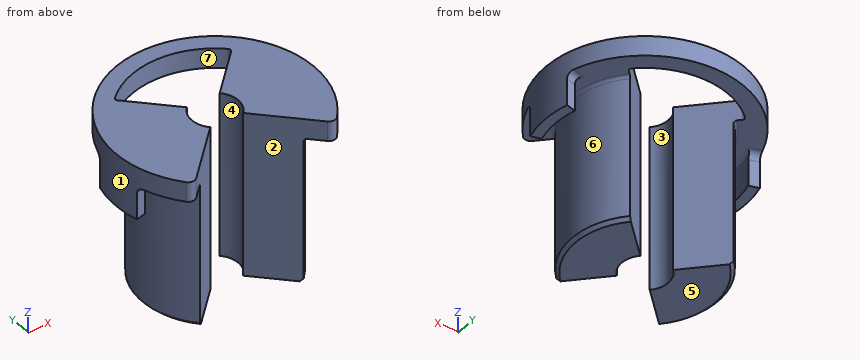
from build123d import *

# Parameters (mm, degrees)
F0_R      = 11
F0_R_2    = 3.5
F1_DEPTH  = 25
F2_R      = 15
F2_R_2    = 3.5
F3_DEPTH  = 8
F4_R      = 13.5
F4_R_2    = 11
F5_DEPTH  = 5
F6_R      = 0.4
F8_DEPTH  = 25
F10_DEPTH = 5
F12_R     = 1
F13_SIZE  = 0.5
F15_DEPTH = 3
F16_R     = 0.4


# Not quite as in the source:
# - a feature of the source that left no trace in its solid (it failed there, or was rolled back) is left out


with BuildPart() as f1:
    # F0 (on Top) → F1 (new body)
    with BuildSketch(Plane.XY):
        Circle(F0_R)
        Circle(F0_R_2, mode=Mode.SUBTRACT)
    extrude(amount=-F1_DEPTH)

    # F2 (on Top) → F3 (join)
    with BuildSketch(Plane.XY):
        Circle(F2_R)
        Circle(F2_R_2, mode=Mode.SUBTRACT)
    extrude(amount=-F3_DEPTH)

    # F4 (on face) → F5 (cut)
    with BuildSketch(Plane(origin=(0, 0, -8), x_dir=(1, 0, 0), z_dir=(0, 0, -1))):
        Circle(F4_R)
        Circle(F4_R_2, mode=Mode.SUBTRACT)
    extrude(amount=-F5_DEPTH, mode=Mode.SUBTRACT)

    # F6
    f6_edges = [f1.edges().sort_by_distance(p)[0] for p in [
        (-13.5, 0, -3),
    ]]
    fillet(f6_edges, radius=F6_R)

    # F7 (on Top) → F8 (cut)
    with BuildSketch(Plane.XY):
        with BuildLine():
            ThreePointArc((-2.4748737342, 2.4748737342), (0, 3.5), (2.4748737342, 2.4748737342))
            Line((2.4748737342, 2.4748737342), (10.6066017178, 10.6066017178))
            ThreePointArc((10.6066017178, 10.6066017178), (0, 15), (-10.6066017178, 10.6066017178))
            Line((-10.6066017178, 10.6066017178), (-2.4748737342, 2.4748737342))
        make_face()
        with BuildLine():
            Line((10.6066017178, -10.6066017178), (2.4748737342, -2.4748737342))
            ThreePointArc((2.4748737342, -2.4748737342), (0, -3.5), (-2.4748737342, -2.4748737342))
            Line((-2.4748737342, -2.4748737342), (-10.6066017178, -10.6066017178))
            ThreePointArc((-10.6066017178, -10.6066017178), (0, -15), (10.6066017178, -10.6066017178))
        make_face()
    extrude(amount=-F8_DEPTH, mode=Mode.SUBTRACT)

    # F9 (on face) → F10 (cut, through all)
    with BuildSketch(Plane(origin=(0, 0, -8), x_dir=(1, 0, 0), z_dir=(0, 0, -1))):
        with BuildLine():
            ThreePointArc((-10.6251840892, 2.8470094961), (0, 11), (10.6251840892, 2.8470094961))
            Line((10.6251840892, 2.8470094961), (15.4548132206, 4.1411047216))
            ThreePointArc((15.4548132206, 4.1411047216), (0, 16), (-15.4548132206, 4.1411047216))
            Line((-15.4548132206, 4.1411047216), (-10.6251840892, 2.8470094961))
        make_face()
        with BuildLine():
            Line((15.4548132206, -4.1411047216), (10.6251840892, -2.8470094961))
            ThreePointArc((10.6251840892, -2.8470094961), (0, -11), (-10.6251840892, -2.8470094961))
            Line((-10.6251840892, -2.8470094961), (-15.4548132206, -4.1411047216))
            ThreePointArc((-15.4548132206, -4.1411047216), (0, -16), (15.4548132206, -4.1411047216))
        make_face()
    extrude(amount=-F10_DEPTH, mode=Mode.SUBTRACT)

    # F12 (call 1 of 6: OpenCascade refuses the feature's edges together)
    f12_edges = [f1.edges().sort_by_distance(p)[0] for p in [
        (10.606602, -10.606602, -1.5),
    ]]
    fillet(f12_edges, radius=F12_R)

    # F12#2 (call 2 of 6)
    f12_2_edges = [f1.edges().sort_by_distance(p)[0] for p in [
        (-10.606602, -10.606602, -1.5),
    ]]
    fillet(f12_2_edges, radius=F12_R)

    # F12#3 (call 3 of 6)
    f12_3_edges = [f1.edges().sort_by_distance(p)[0] for p in [
        (13.571258, -3.636408, -3),
    ]]
    fillet(f12_3_edges, radius=F12_R)

    # F12#4 (call 4 of 6)
    f12_4_edges = [f1.edges().sort_by_distance(p)[0] for p in [
        (13.571258, 3.636408, -3),
    ]]
    fillet(f12_4_edges, radius=F12_R)

    # F12#5 (call 5 of 6)
    f12_5_edges = [f1.edges().sort_by_distance(p)[0] for p in [
        (-13.571258, -3.636408, -3),
    ]]
    fillet(f12_5_edges, radius=F12_R)

    # F12#6 (call 6 of 6)
    f12_6_edges = [f1.edges().sort_by_distance(p)[0] for p in [
        (-13.571258, 3.636408, -3),
    ]]
    fillet(f12_6_edges, radius=F12_R)

    # F13
    f13_edges = [f1.edges().sort_by_distance(p)[0] for p in [
        (-11, 0, -25),
        (11, 0, -25),
    ]]
    chamfer(f13_edges, length=F13_SIZE)

    # F14 (on Top) → F15 (join)
    with BuildSketch(Plane.XY):
        with BuildLine():
            Line((12.5, 0), (15, 0))
            ThreePointArc((15, 0), (0, 15), (-15, 0))
            Line((-15, 0), (-12.5, 0))
            ThreePointArc((-12.5, 0), (0, 12.5), (12.5, 0))
        make_face()
    extrude(amount=-F15_DEPTH)

    # F16
    f16_edges = [f1.edges().sort_by_distance(p)[0] for p in [
        (11, 0, -3),
        (-11, 0, -3),
        (-8.838835, 8.838835, -1.5),
        (8.838835, 8.838835, -1.5),
    ]]
    fillet(f16_edges, radius=F16_R)


solid = f1.part
Build history of the part. All positions in model axes, mm. Face numbers are marked on the shaded views. A direction names the side the tool comes from. Round coordinates to 2 decimals unless told otherwise and drop trailing zeros. Write each loop counter-clockwise with the first axis right and the second up, starting at its lowest first coordinate (ties: lowest second). Pieces come first, ordered by that corner, then holes. Notation, with made-up numbers: M -5,3 L 12,3 A30 cw 12,42 Z; hole C 88,-29.5 d9. An arc over 180 degrees is marked long. Answer in a Markdown table with one row per item.
1. Saw through at B-B (z = -19.5). List the corners of the cut face in (x, y).
Geometry check:
| item | result |
|---|---|
| outline | M -7.78,-7.78 L -2.47,-2.47 A3.5 cw -2.47,2.47 L -7.78,7.78 A11 ccw Z; M 2.47,-2.47 L 7.78,-7.78 A11 ccw 7.78,7.78 L 2.47,2.47 A3.5 cw Z |
2. Saw through at A-A (z = -6.25). List the corners of the cut face in (x, y), and give its area (3 significant figures).
Geometry check:
| item | result |
|---|---|
| outline | M -14.49,-3.88 L -13.04,-3.49 A13.5 cw -13.04,3.49 L -14.49,3.88 A15 ccw Z; M -7.78,-7.78 L -2.47,-2.47 A3.5 cw -2.47,2.47 L -7.78,7.78 A11 ccw Z; M 2.47,-2.47 L 7.78,-7.78 A11 ccw 7.78,7.78 L 2.47,2.47 A3.5 cw Z; M 13.04,-3.49 L 14.49,-3.88 A15 ccw 14.49,3.88 L 13.04,3.49 A13.5 cw Z |
| area | 193 mm2 |
3. Mould opens along Y. For the marked faces 1, 2, 3 and 4 say: +Y half, -Y half, draft (parallel to the pull), parting line (faces both ways), or undercut.
Geometry check:
| item | result |
|---|---|
| face 1 | parting line |
| face 2 | -Y half |
| face 3 | undercut |
| face 4 | undercut |
4. Flat gauge pins, fed straight in: P1, Ø4, axis at x = -0.5, y = 4.5, coming from the -Z side; P2, Ø12, axis at x = 9, z = -20.5, coming from the +Y side; P3, Ø2, axis at x = 5, z = -13.5, coming from the +Y side; P4, Ø2, axis at x = 14.5, y = 0.5, coming from the -Z side. Where does each tip first touch, or does it go through?
Geometry check:
| item | result |
|---|---|
| P1 | through |
| P2 | y = 7.78 |
| P3 | y = 6 |
| P4 | z = -8 |
5. Saw through at C-C (y = 0). List the corners of the cut face in (x, z), and give its area (3 significant figures).
Geometry check:
| item | result |
|---|---|
| outline | M -15,-8 L -13.5,-8 L -13.5,-3.4 A0.4 cw -13.1,-3 L -11.4,-3 A0.4 cw -11,-3.4 L -11,-24.5 L -10.5,-25 L -3.5,-25 L -3.5,0 L -15,0 Z; M 3.5,-25 L 10.5,-25 L 11,-24.5 L 11,-3.4 A0.4 cw 11.4,-3 L 13.1,-3 A0.4 cw 13.5,-3.4 L 13.5,-8 L 15,-8 L 15,0 L 3.5,0 Z |
| area | 414 mm2 |
6. Which spindle directions (+Z, -Z, +X, -X, +Y, -Y) get a long thin tool onto all of the face, cutting with end or side? Do the marked faces 5, 6 and 7. Say none if no direction does.
Geometry check:
| item | result |
|---|---|
| face 5 | -Z, +X, -X, +Y, -Y |
| face 6 | -Z |
| face 7 | +Z, -Z |
7. Probe L1, parallel to X at y = -2.25, z = -6.5; L2, parallel to Z at x = -4.5, y = 12; L3, parallel to X at y = -2.75, z = -21. List the from-to ranges inside material, lowest first. Write a range as [from, to].
Geometry check:
| item | result |
|---|---|
| L1 | [-14.83, -13.31], [-10.77, -2.68], [2.68, 10.77], [13.31, 14.83] |
| L2 | [-3, 0] |
| L3 | [-10.65, -2.75], [2.75, 10.65] |
8. Saw through at D-D (x = 7). List the corners of the cut face in (y, z).
Geometry check:
| item | result |
|---|---|
| outline | M -7,-25 L 7,-25 L 7,0 L -7,0 Z; M 10.36,-3 L 13.27,-3 L 13.27,0 L 10.36,0 Z |
